Part model, mm, in its own coordinate system. Give positions to 0.01 mm unless a question says otherwise; leave off trailing zeros. Write each question's results on one line, items separated by ' | '. Start each with the question number.
from build123d import *

# Parameters (mm, degrees)
F0_W     = 178
F0_H     = 178
F0_R     = 8.3
F1_DEPTH = 3.2
F2_W     = 178
F2_H     = 178
F3_DEPTH = 9.5


with BuildPart() as f1:
    # F0 (on Top) → F1 (new body)
    with BuildSketch(Plane.XY):
        with Locations((78.75, 78.75)):
            Rectangle(F0_W, F0_H)
        Circle(F0_R, mode=Mode.SUBTRACT)
        with Locations((17.5, 0)):
            Circle(F0_R, mode=Mode.SUBTRACT)
        with Locations((0, 17.5)):
            Circle(F0_R, mode=Mode.SUBTRACT)
        with Locations((17.5, 17.5)):
            Circle(F0_R, mode=Mode.SUBTRACT)
        with Locations((35, 0)):
            Circle(F0_R, mode=Mode.SUBTRACT)
        with Locations((52.5, 0)):
            Circle(F0_R, mode=Mode.SUBTRACT)
        with Locations((70, 0)):
            Circle(F0_R, mode=Mode.SUBTRACT)
        with Locations((35, 17.5)):
            Circle(F0_R, mode=Mode.SUBTRACT)
        with Locations((52.5, 17.5)):
            Circle(F0_R, mode=Mode.SUBTRACT)
        with Locations((70, 17.5)):
            Circle(F0_R, mode=Mode.SUBTRACT)
        with Locations((0, 35)):
            Circle(F0_R, mode=Mode.SUBTRACT)
        with Locations((0, 52.5)):
            Circle(F0_R, mode=Mode.SUBTRACT)
        with Locations((17.5, 35)):
            Circle(F0_R, mode=Mode.SUBTRACT)
        with Locations((17.5, 52.5)):
            Circle(F0_R, mode=Mode.SUBTRACT)
        with Locations((0, 70)):
            Circle(F0_R, mode=Mode.SUBTRACT)
        with Locations((17.5, 70)):
            Circle(F0_R, mode=Mode.SUBTRACT)
        with Locations((35, 35)):
            Circle(F0_R, mode=Mode.SUBTRACT)
        with Locations((52.5, 35)):
            Circle(F0_R, mode=Mode.SUBTRACT)
        with Locations((35, 52.5)):
            Circle(F0_R, mode=Mode.SUBTRACT)
        with Locations((52.5, 52.5)):
            Circle(F0_R, mode=Mode.SUBTRACT)
        with Locations((70, 35)):
            Circle(F0_R, mode=Mode.SUBTRACT)
        with Locations((70, 52.5)):
            Circle(F0_R, mode=Mode.SUBTRACT)
        with Locations((35, 70)):
            Circle(F0_R, mode=Mode.SUBTRACT)
        with Locations((52.5, 70)):
            Circle(F0_R, mode=Mode.SUBTRACT)
        with Locations((70, 70)):
            Circle(F0_R, mode=Mode.SUBTRACT)
        with Locations((87.5, 0)):
            Circle(F0_R, mode=Mode.SUBTRACT)
        with Locations((105, 0)):
            Circle(F0_R, mode=Mode.SUBTRACT)
        with Locations((122.5, 0)):
            Circle(F0_R, mode=Mode.SUBTRACT)
        with Locations((87.5, 17.5)):
            Circle(F0_R, mode=Mode.SUBTRACT)
        with Locations((105, 17.5)):
            Circle(F0_R, mode=Mode.SUBTRACT)
        with Locations((122.5, 17.5)):
            Circle(F0_R, mode=Mode.SUBTRACT)
        with Locations((140, 0)):
            Circle(F0_R, mode=Mode.SUBTRACT)
        with Locations((157.5, 0)):
            Circle(F0_R, mode=Mode.SUBTRACT)
        with Locations((140, 17.5)):
            Circle(F0_R, mode=Mode.SUBTRACT)
        with Locations((157.5, 17.5)):
            Circle(F0_R, mode=Mode.SUBTRACT)
        with Locations((87.5, 35)):
            Circle(F0_R, mode=Mode.SUBTRACT)
        with Locations((87.5, 52.5)):
            Circle(F0_R, mode=Mode.SUBTRACT)
        with Locations((105, 35)):
            Circle(F0_R, mode=Mode.SUBTRACT)
        with Locations((122.5, 35)):
            Circle(F0_R, mode=Mode.SUBTRACT)
        with Locations((105, 52.5)):
            Circle(F0_R, mode=Mode.SUBTRACT)
        with Locations((122.5, 52.5)):
            Circle(F0_R, mode=Mode.SUBTRACT)
        with Locations((87.5, 70)):
            Circle(F0_R, mode=Mode.SUBTRACT)
        with Locations((105, 70)):
            Circle(F0_R, mode=Mode.SUBTRACT)
        with Locations((122.5, 70)):
            Circle(F0_R, mode=Mode.SUBTRACT)
        with Locations((140, 35)):
            Circle(F0_R, mode=Mode.SUBTRACT)
        with Locations((140, 52.5)):
            Circle(F0_R, mode=Mode.SUBTRACT)
        with Locations((157.5, 35)):
            Circle(F0_R, mode=Mode.SUBTRACT)
        with Locations((157.5, 52.5)):
            Circle(F0_R, mode=Mode.SUBTRACT)
        with Locations((140, 70)):
            Circle(F0_R, mode=Mode.SUBTRACT)
        with Locations((157.5, 70)):
            Circle(F0_R, mode=Mode.SUBTRACT)
        with Locations((0, 87.5)):
            Circle(F0_R, mode=Mode.SUBTRACT)
        with Locations((17.5, 87.5)):
            Circle(F0_R, mode=Mode.SUBTRACT)
        with Locations((0, 105)):
            Circle(F0_R, mode=Mode.SUBTRACT)
        with Locations((0, 122.5)):
            Circle(F0_R, mode=Mode.SUBTRACT)
        with Locations((17.5, 105)):
            Circle(F0_R, mode=Mode.SUBTRACT)
        with Locations((17.5, 122.5)):
            Circle(F0_R, mode=Mode.SUBTRACT)
        with Locations((35, 87.5)):
            Circle(F0_R, mode=Mode.SUBTRACT)
        with Locations((52.5, 87.5)):
            Circle(F0_R, mode=Mode.SUBTRACT)
        with Locations((70, 87.5)):
            Circle(F0_R, mode=Mode.SUBTRACT)
        with Locations((35, 105)):
            Circle(F0_R, mode=Mode.SUBTRACT)
        with Locations((52.5, 105)):
            Circle(F0_R, mode=Mode.SUBTRACT)
        with Locations((35, 122.5)):
            Circle(F0_R, mode=Mode.SUBTRACT)
        with Locations((52.5, 122.5)):
            Circle(F0_R, mode=Mode.SUBTRACT)
        with Locations((70, 105)):
            Circle(F0_R, mode=Mode.SUBTRACT)
        with Locations((70, 122.5)):
            Circle(F0_R, mode=Mode.SUBTRACT)
        with Locations((0, 140)):
            Circle(F0_R, mode=Mode.SUBTRACT)
        with Locations((17.5, 140)):
            Circle(F0_R, mode=Mode.SUBTRACT)
        with Locations((0, 157.5)):
            Circle(F0_R, mode=Mode.SUBTRACT)
        with Locations((17.5, 157.5)):
            Circle(F0_R, mode=Mode.SUBTRACT)
        with Locations((35, 140)):
            Circle(F0_R, mode=Mode.SUBTRACT)
        with Locations((52.5, 140)):
            Circle(F0_R, mode=Mode.SUBTRACT)
        with Locations((70, 140)):
            Circle(F0_R, mode=Mode.SUBTRACT)
        with Locations((35, 157.5)):
            Circle(F0_R, mode=Mode.SUBTRACT)
        with Locations((52.5, 157.5)):
            Circle(F0_R, mode=Mode.SUBTRACT)
        with Locations((70, 157.5)):
            Circle(F0_R, mode=Mode.SUBTRACT)
        with Locations((87.5, 87.5)):
            Circle(F0_R, mode=Mode.SUBTRACT)
        with Locations((105, 87.5)):
            Circle(F0_R, mode=Mode.SUBTRACT)
        with Locations((122.5, 87.5)):
            Circle(F0_R, mode=Mode.SUBTRACT)
        with Locations((87.5, 105)):
            Circle(F0_R, mode=Mode.SUBTRACT)
        with Locations((87.5, 122.5)):
            Circle(F0_R, mode=Mode.SUBTRACT)
        with Locations((105, 105)):
            Circle(F0_R, mode=Mode.SUBTRACT)
        with Locations((122.5, 105)):
            Circle(F0_R, mode=Mode.SUBTRACT)
        with Locations((105, 122.5)):
            Circle(F0_R, mode=Mode.SUBTRACT)
        with Locations((122.5, 122.5)):
            Circle(F0_R, mode=Mode.SUBTRACT)
        with Locations((140, 87.5)):
            Circle(F0_R, mode=Mode.SUBTRACT)
        with Locations((157.5, 87.5)):
            Circle(F0_R, mode=Mode.SUBTRACT)
        with Locations((140, 105)):
            Circle(F0_R, mode=Mode.SUBTRACT)
        with Locations((140, 122.5)):
            Circle(F0_R, mode=Mode.SUBTRACT)
        with Locations((157.5, 105)):
            Circle(F0_R, mode=Mode.SUBTRACT)
        with Locations((157.5, 122.5)):
            Circle(F0_R, mode=Mode.SUBTRACT)
        with Locations((87.5, 140)):
            Circle(F0_R, mode=Mode.SUBTRACT)
        with Locations((105, 140)):
            Circle(F0_R, mode=Mode.SUBTRACT)
        with Locations((122.5, 140)):
            Circle(F0_R, mode=Mode.SUBTRACT)
        with Locations((87.5, 157.5)):
            Circle(F0_R, mode=Mode.SUBTRACT)
        with Locations((105, 157.5)):
            Circle(F0_R, mode=Mode.SUBTRACT)
        with Locations((122.5, 157.5)):
            Circle(F0_R, mode=Mode.SUBTRACT)
        with Locations((140, 140)):
            Circle(F0_R, mode=Mode.SUBTRACT)
        with Locations((157.5, 140)):
            Circle(F0_R, mode=Mode.SUBTRACT)
        with Locations((140, 157.5)):
            Circle(F0_R, mode=Mode.SUBTRACT)
        with Locations((157.5, 157.5)):
            Circle(F0_R, mode=Mode.SUBTRACT)
    extrude(amount=F1_DEPTH)

    # F2 (on Top) → F3 (join)
    with BuildSketch(Plane.XY):
        with Locations((78.75, 78.75)):
            Rectangle(F2_W, F2_H)
    extrude(amount=-F3_DEPTH)


solid = f1.part
(1) Pull direction X, two halves, no side cores. Call faces 1 (the flat face through (-10.25, 78, -3)), 2 (the cylindrical face through (109.46, 112, 1.58)): +X half, -X half, draft (parallel to the pull), parting line (faces both ways), or undercut.
(2) Drop flat-ended pins along their axis: P1, Ø19, axis at x = 157.5, y = 157.5, coming from the +Z side; P2, Ø1, axis at x = 50.5, y = 77, coming from the +Z side. Give the stop position or say it passes through.
(3) Probe L1, parallel to Z at x = 102.5, y = 83.5. List the from-to ranges inside material, lowest first.
Taken from the geometry:
1) face 1: -X half | face 2: undercut
2) P1: stops at z = 3.2 | P2: stops at z = 0
3) L1: z = -9.5 to 0
